Can you work these out from the drawing? Everything is in mm from the part's minimum corner. A direction names the side the tool comes from. Round coordinates to 2 decimals unless told otherwise and drop trailing zeros. Write each loop counter-clockwise with the first axis right and the second up, starting at its lowest first coordinate (ties: lowest second). Pieces come first, ordered by that corner, then holes. Notation, with made-up numbers: (16, 16) - (70, 16) arc R30 cw to (70, 39) - close; hole circle Ø3 at (-19, -8.75). An arc over 180 degrees is marked (long way). One line per item, written item: value. Start each with the question number.
Item 1: For the marked faces 1 and 2, which set-ups out of +Z, -Z, +X, -X, +Y, -Y let a thin tool reach every point of the face, with its end or its side?
Item 2: Imagine slicing it at C-C, the plane z = 7.5. Please give me the cut outline in (x, y), then the cut area to 3 significant figures.
Item 3: For P1, Ø1, axis at x = 3, z = 10.5, coming from the -Y side; P2, Ø6, axis at y = 46.5, z = 4, coming from the -X side; P3, Ø2, axis at x = 2, y = 51.5, coming from the -Z side; P4, Ø2, axis at x = 3, y = 52.5, coming from the +Z side, each with a flat end and sliding along its axis, tell me the tip position at first contact or that it passes through.
Item 4: Imagine slicing it at D-D, the plane y = 31.5. Please give me the cut outline in (x, z).
Item 5: Imagine slicing it at A-A, the plane y = 50.5. Please give me the cut outline in (x, z).
Item 6: Thinking about a two-plate mould opening in Y: for the marked faces 3, 4 and 5, which applies, released by +Y, released by -Y, zero draft, split by the parting line, or undercut?
Item 7: Imagine slicing it at B-B, the plane x = 3.3. Please give me the cut outline in (y, z), then the cut area to 3 significant figures.
Item 8: If I drill on line 1 (Y direction, x = 1, z = 8); line 2 (Z direction, x = 1.35, y = 10); line 3 (Y direction, x = 1.3, z = 6.5), over which ranges is the centre line in solid material (lowest first)?
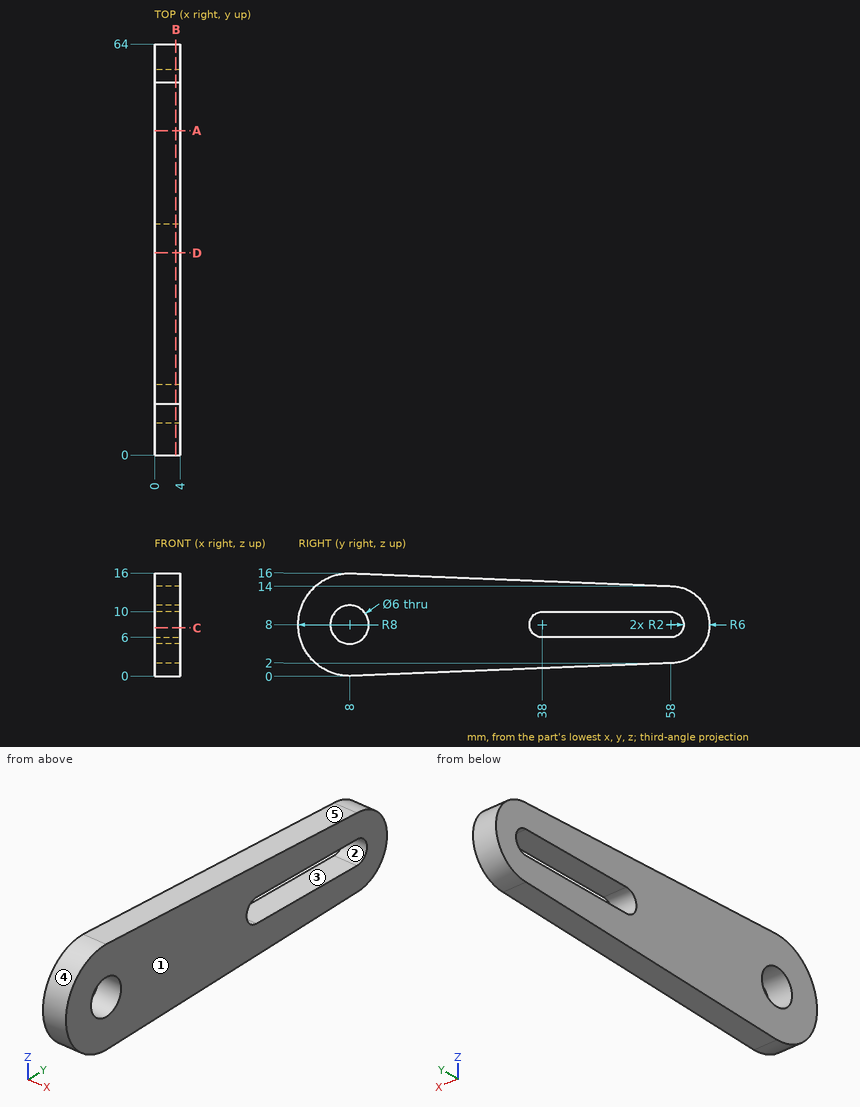
Values follow:
1. face 1: +Z, -Z, +X, +Y, -Y
1. face 2: +X, -X
2. outline: (0, 0.02) - (4, 0.02) - (4, 5.04) - (0, 5.04) - close; (0, 10.96) - (4, 10.96) - (4, 36.06) - (0, 36.06) - close; (0, 59.94) - (4, 59.94) - (4, 63.98) - (0, 63.98) - close
2. area: 137 mm^2
3. P1: stops at y = 0.25
3. P2: stops at x = 0
3. P3: stops at z = 1.7
3. P4: stops at z = 14.26
4. outline: (0, 0.94) - (4, 0.94) - (4, 15.06) - (0, 15.06) - close
5. outline: (0, 1.7) - (4, 1.7) - (4, 6) - (0, 6) - close; (0, 10) - (4, 10) - (4, 14.3) - (0, 14.3) - close
6. face 3: undercut
6. face 4: released by -Y
6. face 5: released by +Y
7. outline: (8, 0) - (58, 2) arc R6 ccw to (58, 14) - (8, 16) arc R8 ccw to start; hole circle Ø6 at (8, 8); hole (38, 6) - (58, 6) arc R2 ccw to (58, 10) - (38, 10) arc R2 ccw to start
7. area: 736 mm^2
8. line 1: y = 0 to 5, 11 to 36, 60 to 64
8. line 2: z = 0.08 to 5.76, 10.24 to 15.92
8. line 3: y = 0.14 to 5.4, 10.6 to 36.68, 59.32 to 63.81
